Input: part model. Units: mm. Frame: model coordinates. Face numbers are marked on the shaded views. A direction names the side the tool comes from. Coordinates: 2 decimals unless noted, no trailing zeros. Loops run counter-clockwise (first coordinate to the right, second up) from the corner with the lowest first, then second, coordinate; pieces in that order, holes last.
Item 1: Reachability of the marked faces 1, 2 and 3 from +Z, -Z, +X, -X, +Y, -Y: full face, straight path, thin tool, end or side. Return the list, or none.
Item 2: Section B-B on z = 113.5. Return loops of the section in (x, y), and give its area (3 significant figures).
Item 3: Contact query for flat-ended pins moving along their axis: P1, Ø19.5, axis at x = 6.5, z = 35.5, coming from the -Y side; P2, Ø3, axis at x = -14.5, y = -48, coming from the -Z side; P3, Ø1, axis at x = -30.5, y = -8.5, coming from the +Z side. Output: stop coordinate, or through.
Item 4: Pull-direction query (X, two-part tool) for the marked faces 4, 5 and 6; classes: released by +X, released by -X, zero draft, split by the parting line, or undercut.
Item 5: Section C-C on y = 18. Return loops of the section in (x, z).
Item 6: Ray query, line 1 along Y through (x, z) = (-33, 71.5); line 2 along X through (y, z) = (-23.5, 173); line 3 along Z through (x, y) = (35, -16). Return the intervals inside material, ascending.
Item 7: Section A-A on x = -31.5. Return loops of the section in (y, z).
```python
from build123d import *

# Parameters (mm, degrees)
F0_W     = 88.061482
F0_H     = 88.219233
F1_DEPTH = 182.118
F2_W     = 75.133953
F2_H     = 74.157518
F3_DEPTH = 175.26
F4_W     = 81.089504
F4_H     = 6.89533
F5_DEPTH = 183.134
F6_W     = 6.971978
F6_H     = 6.89533
F7_DEPTH = 187.706
F8_W     = 81.089504
F8_H     = 10.767195
F8_W_2   = 6.971978
F9_DEPTH = 117.094


with BuildPart() as f1:
    # F0 (on Top) → F1 (new body)
    with BuildSketch(Plane.XY):
        with Locations((2.006993, -2.8916)):
            Rectangle(F0_W, F0_H)
    extrude(amount=F1_DEPTH)

    # F2 (on face) → F3 (cut)
    with BuildSketch(Plane.XY.offset(182.118)):
        with Locations((1.49878, -3.027128)):
            Rectangle(F2_W, F2_H)
    extrude(amount=-F3_DEPTH, mode=Mode.SUBTRACT)

    # F4 (on face) → F5 (cut)
    with BuildSketch(Plane.XY.offset(182.118)):
        with Locations((-1.478996, -43.553552)):
            Rectangle(F4_W, F4_H)
    extrude(amount=-F5_DEPTH, mode=Mode.SUBTRACT)

    # F6 (on face) → F7 (cut)
    with BuildSketch(Plane(origin=(0, 0, 0), x_dir=(1, 0, 0), z_dir=(0, 0, -1))):
        with Locations((42.551745, 43.553552)):
            Rectangle(F6_W, F6_H)
    extrude(amount=-F7_DEPTH, mode=Mode.SUBTRACT)

    # F8 (on face) → F9 (join)
    with BuildSketch(Plane.XY.offset(182.118)):
        with Locations((-1.478996, -45.489484)):
            Rectangle(F8_W, F8_H)
        with Locations((42.551745, -45.489484)):
            Rectangle(F8_W_2, F8_H)
    extrude(amount=-F9_DEPTH)


solid = f1.part
```
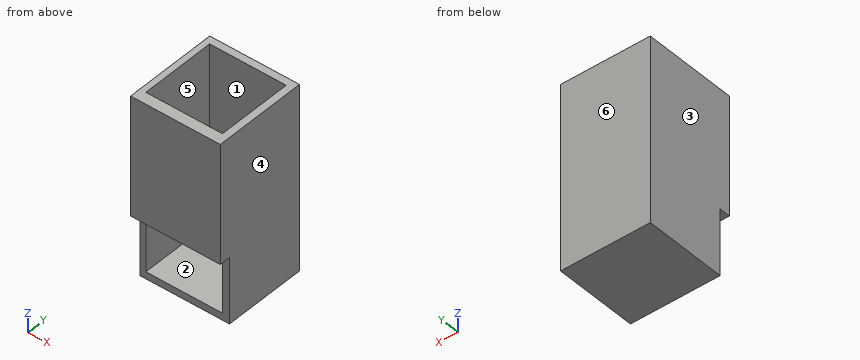
Results found:
1. face 1: +Z
1. face 2: +Z, -Y
1. face 3: +Z, -Z, -X, +Y, -Y
2. outline: (-42.02, -50.87) - (46.04, -50.87) - (46.04, 41.22) - (-42.02, 41.22) - close; hole (-36.07, -40.11) - (39.07, -40.11) - (39.07, 34.05) - (-36.07, 34.05) - close
2. area: 2,540 mm2
3. P1: stops at y = 34.05
3. P2: stops at z = 65.02
3. P3: stops at z = 6.86
4. face 4: released by +X
4. face 5: undercut
4. face 6: zero draft
5. outline: (-42.02, 0) - (46.04, 0) - (46.04, 182.12) - (39.07, 182.12) - (39.07, 6.86) - (-36.07, 6.86) - (-36.07, 182.12) - (-42.02, 182.12) - close
6. line 1: y = -50.87 to -40.11, 34.05 to 41.22
6. line 2: x = -42.02 to -36.07, 39.07 to 46.04
6. line 3: z = 0 to 6.86
7. outline: (-50.87, 65.02) - (-40.11, 65.02) - (-40.11, 182.12) - (-50.87, 182.12) - close; (-40.11, 0) - (41.22, 0) - (41.22, 182.12) - (34.05, 182.12) - (34.05, 6.86) - (-40.11, 6.86) - close
